Verification items for the finished model (mm, model axes). Face numbers are marked on the shaded views. A direction names the side the tool comes from. Round coordinates to 2 decimals unless told otherwise and drop trailing zeros. Write each loop counter-clockwise with the first axis right and the second up, starting at its lowest first coordinate (ties: lowest second). Pieces come first, ordered by that corner, then holes. Notation, with made-up numbers: M 22,-3 L 45,-3 A9 cw 45,3 Z; hole C 63,-6.75 d6. An arc over 180 degrees is marked long. One line per item, written item: value. Start each with the question number.
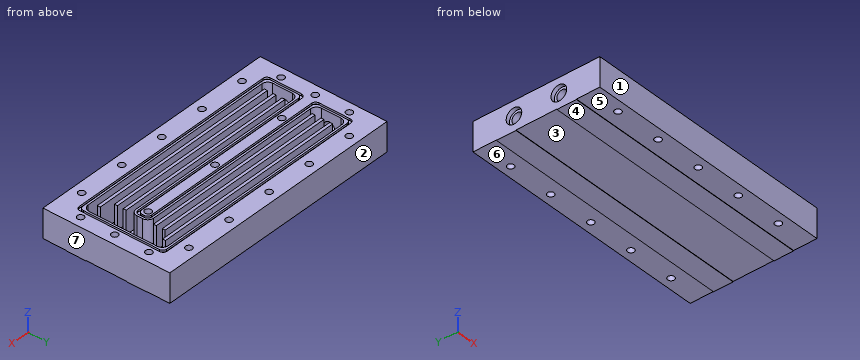
from build123d import *

# Parameters (mm, degrees)
ESQUISSE1_W             = 130
ESQUISSE1_H             = 65
BOSS_EXTRU_1_DEPTH      = 14.8
ESQUISSE13_W            = 130
ESQUISSE13_H            = 10
BOSS_EXTRU_3_DEPTH      = 0.2
D_GAGEMENT_M31_D        = 3.4
ENL_V_MAT_EXTRU_6_DEPTH = 12
D_GAGEMENT_M51_D        = 5.5
D_GAGEMENT_M51_DEPTH    = 10
ESQUISSE10_R            = 4
ENL_V_MAT_EXTRU_7_DEPTH = 2
ENL_V_MAT_EXTRU_9_DEPTH = 1
ESQUISSE12_W            = 100
ESQUISSE12_H            = 1.5
ESQUISSE12_W_2          = 95
BOSS_EXTRU_2_DEPTH      = 12
D_GAGEMENT_M32_D        = 3.4
D_GAGEMENT_M32_DEPTH    = 8.978536948
D_GAGEMENT_M32_TIP      = 1.021463052


with BuildPart() as part:
    # Esquisse1 → Boss.-Extru.1 (new body)
    with BuildSketch(Plane.XY):
        with Locations((65, 32.5)):
            Rectangle(ESQUISSE1_W, ESQUISSE1_H)
    extrude(amount=BOSS_EXTRU_1_DEPTH)

    # Esquisse13 → Boss.-Extru.3 (add)
    with BuildSketch(Plane(origin=(0, 0, 0), x_dir=(-1, 0, 0), z_dir=(0, 0, -1))):
        with Locations((-65, 48)):
            Rectangle(ESQUISSE13_W, ESQUISSE13_H)
        with Locations((-65, 17)):
            Rectangle(ESQUISSE13_W, ESQUISSE13_H)
    extrude(amount=BOSS_EXTRU_3_DEPTH)

    # Dégagement M31 (through all)
    with Locations(Plane.XY.offset(14.8)):
        with Locations((16.7, 60), (40.7, 60), (64.7, 60), (88.7, 60), (112.7, 60), (112.7, 5), (88.7, 5), (64.7, 5), (40.7, 5), (16.7, 5)):
            Hole(D_GAGEMENT_M31_D / 2)

    # Esquisse6 → Enlèv. mat.-Extru.6 (cut)
    with BuildSketch(Plane.XY.offset(14.8)):
        with BuildLine():
            Line((13, 53), (117, 53))
            ThreePointArc((117, 53), (119.121320344, 52.121320344), (120, 50))
            Line((120, 50), (120, 15))
            ThreePointArc((120, 15), (119.121320344, 12.878679656), (117, 12))
            Line((117, 12), (13, 12))
            ThreePointArc((13, 12), (10.878679656, 12.878679656), (10, 15))
            Line((10, 15), (10, 25))
            ThreePointArc((10, 25), (10.878679656, 27.121320344), (13, 28))
            Line((13, 28), (107, 28))
            ThreePointArc((107, 28), (109.121320344, 28.878679656), (110, 31))
            Line((110, 31), (110, 34))
            ThreePointArc((110, 34), (109.121320344, 36.121320344), (107, 37))
            Line((107, 37), (13, 37))
            ThreePointArc((13, 37), (10.878679656, 37.878679656), (10, 40))
            Line((10, 40), (10, 50))
            ThreePointArc((10, 50), (10.878679656, 52.121320344), (13, 53))
        make_face()
    extrude(amount=-ENL_V_MAT_EXTRU_6_DEPTH, mode=Mode.SUBTRACT)

    # Dégagement M51
    with Locations(Plane.ZY):
        with Locations((7.3, 44), (7.3, 21)):
            Hole(D_GAGEMENT_M51_D / 2, depth=D_GAGEMENT_M51_DEPTH)

    # Esquisse10 → Enlèv. mat.-Extru.7 (cut)
    with BuildSketch(Plane.ZY):
        with Locations((7.3, 21)):
            Circle(ESQUISSE10_R)
        with Locations((7.3, 44)):
            Circle(ESQUISSE10_R)
    extrude(amount=-ENL_V_MAT_EXTRU_7_DEPTH, mode=Mode.SUBTRACT)

    # Esquisse11 → Enlèv. mat.-Extru.9 (cut)
    with BuildSketch(Plane.XY.offset(14.8)):
        with BuildLine():
            Line((120, 10), (10, 10))
            ThreePointArc((10, 10), (8.585786438, 10.585786438), (8, 12))
            Line((8, 12), (8, 28))
            ThreePointArc((8, 28), (8.585786438, 29.414213562), (10, 30))
            Line((10, 30), (106, 30))
            ThreePointArc((106, 30), (107.414213562, 30.585786438), (108, 32))
            Line((108, 32), (108, 33))
            ThreePointArc((108, 33), (107.414213562, 34.414213562), (106, 35))
            Line((106, 35), (10, 35))
            ThreePointArc((10, 35), (8.585786438, 35.585786438), (8, 37))
            Line((8, 37), (8, 53))
            ThreePointArc((8, 53), (8.585786438, 54.414213562), (10, 55))
            Line((10, 55), (120, 55))
            ThreePointArc((120, 55), (121.414213562, 54.414213562), (122, 53))
            Line((122, 53), (122, 12))
            ThreePointArc((122, 12), (121.414213562, 10.585786438), (120, 10))
        make_face()
        with BuildLine():
            Line((11, 54), (119, 54))
            ThreePointArc((119, 54), (120.414213562, 53.414213562), (121, 52))
            Line((121, 52), (121, 13))
            ThreePointArc((121, 13), (120.414213562, 11.585786438), (119, 11))
            Line((119, 11), (11, 11))
            ThreePointArc((11, 11), (9.585786438, 11.585786438), (9, 13))
            Line((9, 13), (9, 27))
            ThreePointArc((9, 27), (9.585786438, 28.414213562), (11, 29))
            Line((11, 29), (107, 29))
            ThreePointArc((107, 29), (108.414213562, 29.585786438), (109, 31))
            Line((109, 31), (109, 34))
            ThreePointArc((109, 34), (108.414213562, 35.414213562), (107, 36))
            Line((107, 36), (11, 36))
            ThreePointArc((11, 36), (9.585786438, 36.585786438), (9, 38))
            Line((9, 38), (9, 52))
            ThreePointArc((9, 52), (9.585786438, 53.414213562), (11, 54))
        make_face(mode=Mode.SUBTRACT)
    extrude(amount=-ENL_V_MAT_EXTRU_9_DEPTH, mode=Mode.SUBTRACT)

    # Esquisse12 → Boss.-Extru.2 (add)
    with BuildSketch(Plane.XY.offset(2.8)):
        with Locations((65, 15.75)):
            Rectangle(ESQUISSE12_W, ESQUISSE12_H)
        with Locations((62.5, 20.25)):
            Rectangle(ESQUISSE12_W_2, ESQUISSE12_H)
        with Locations((62.5, 24.75)):
            Rectangle(ESQUISSE12_W_2, ESQUISSE12_H)
        with Locations((62.5, 40.25)):
            Rectangle(ESQUISSE12_W_2, ESQUISSE12_H)
        with Locations((62.5, 44.75)):
            Rectangle(ESQUISSE12_W_2, ESQUISSE12_H)
        with Locations((65, 49.25)):
            Rectangle(ESQUISSE12_W, ESQUISSE12_H)
    extrude(amount=BOSS_EXTRU_2_DEPTH)

    # Dégagement M32
    with Locations(Plane.XY.offset(14.8)):
        with Locations((5, 50), (5, 15), (25, 32.5), (65, 32.5), (105, 32.5), (125, 15), (125, 50), (5, 32.5), (125, 32.5)):
            Hole(D_GAGEMENT_M32_D / 2, depth=D_GAGEMENT_M32_DEPTH)
            with Locations((0, 0, -(D_GAGEMENT_M32_DEPTH + D_GAGEMENT_M32_TIP / 2))):  # 118° drill point
                Cone(0, D_GAGEMENT_M32_D / 2, D_GAGEMENT_M32_TIP, mode=Mode.SUBTRACT)


solid = part.part
1) Cross-section at A-A (y = 60). Record the boundary of the cut face in (x, z).
2) Thickness scan on line 1 (X direction, y = 40, z = 4.75); line 2 (Y direction, x = 125, z = 8.5); line 3 (X direction, y = 53.5, z = 14). Record the ranges inside material, lowest first.
3) Access from +Z, -Z, +X, -X, +Y, -Y to the whole of each face (thin tool, end or side, straight path). Record for the marked faces 5, 6 and 7.
4) Cross-section at B-B (z = 8). State how many separate pieces and enclosed holes the cut face has, then the cut area to 3 significant figures.
5) Gauge pin test, flat ends, axial feed: pin 1 Ø9.5 at (x, y) = (72, 5) entering from -Z; pin 2 Ø2.5 at (y, z) = (45, 6.5) entering from -X; pin 3 Ø6.5 at (y, z) = (44, 7.3) entering from -X. Record the tip position at first contact, or that the pin passes through.
6) Mould release check, pull along Y, two halves, no side actions. Record for the marked faces 1, 2, 3 and 4: pulls with the +Y half, pulls with the -Y half, needs draft (parallel to the pull), parting line crosses it, or undercut.
Results below:
1. outline: M 0,0 L 15,0 L 15,14.8 L 0,14.8 Z; M 18.4,0 L 39,0 L 39,14.8 L 18.4,14.8 Z; M 42.4,0 L 63,0 L 63,14.8 L 42.4,14.8 Z; M 66.4,0 L 87,0 L 87,14.8 L 66.4,14.8 Z; M 90.4,0 L 111,0 L 111,14.8 L 90.4,14.8 Z; M 114.4,0 L 130,0 L 130,14.8 L 114.4,14.8 Z
2. line 1: x = 0 to 10, 15 to 110, 120 to 130
2. line 2: y = 0 to 13.3, 16.7 to 30.8, 34.2 to 48.3, 51.7 to 65
2. line 3: x = 0 to 8.06, 9.68 to 120.32, 121.94 to 130
3. face 5: -Z, +X, -X, -Y
3. face 6: -Z, +X, -X, +Y
3. face 7: +Z, -Z, +X, +Y, -Y
4. separate pieces: 8
4. enclosed holes: 19
4. area: 5,430 mm²
5. pin 1: stops at z = 0
5. pin 2: stops at x = 15
5. pin 3: stops at x = 2
6. face 1: pulls with the -Y half
6. face 2: pulls with the +Y half
6. face 3: undercut
6. face 4: needs draft
